Here's how the part is built. I have some questions about the finished solid (model axes, mm). Face numbers are marked on the shaded views. A direction names the side the tool comes from. Give positions to 0.01 mm unless a question says otherwise; leave off trailing zeros. Loops run counter-clockwise (first coordinate to the right, second up) from the corner with the lowest first, then second, coordinate; pieces in that order, holes last. Notation, with made-up numbers: (-15.5, -3.75) - (-2.5, -3.75) arc R36 ccw to (-2.5, 35.25) - close; hole circle Ø1 at (20.25, 40.25). An arc over 180 degrees is marked (long way). One line per item, written item: value. Start each with the question number.
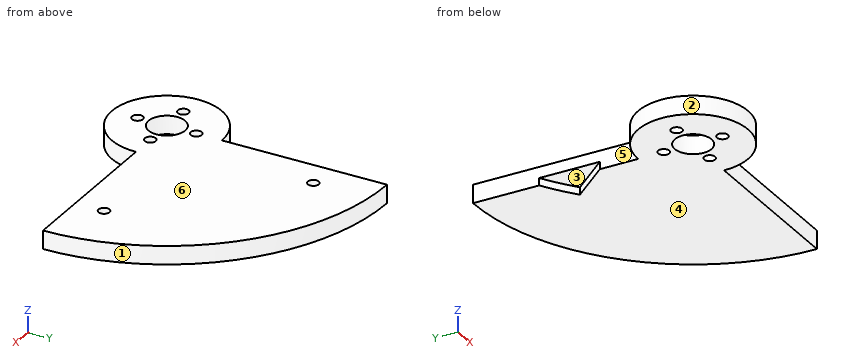
```python
from build123d import *

# Parameters (mm, degrees)
BOSS_EXTRUDE1_DEPTH = 5
SKETCH2_R           = 15
BOSS_EXTRUDE2_DEPTH = 5
SKETCH3_R           = 5
CUT_EXTRUDE1_DEPTH  = 5
SKETCH4_R           = 1.5
CUT_EXTRUDE2_DEPTH  = 2
CUT_EXTRUDE3_DEPTH  = 2
SKETCH6_R           = 1.5
CUT_EXTRUDE4_DEPTH  = 10


with BuildPart() as part:
    # Sketch1 → Boss-Extrude1 (new body)
    with BuildSketch(Plane.XY):
        with BuildLine():
            Line((0, 0), (0, 60))
            ThreePointArc((0, 60), (42.426406871, 42.426406871), (60, 0))
            Line((60, 0), (0, 0))
        make_face()
    extrude(amount=BOSS_EXTRUDE1_DEPTH)

    # Sketch2 → Boss-Extrude2 (add)
    with BuildSketch(Plane.XY.offset(5)):
        Circle(SKETCH2_R)
    extrude(amount=-BOSS_EXTRUDE2_DEPTH)

    # Sketch3 → Cut-Extrude1 (cut)
    with BuildSketch(Plane.XY.offset(5)):
        Circle(SKETCH3_R)
    extrude(amount=-CUT_EXTRUDE1_DEPTH, mode=Mode.SUBTRACT)

    # Sketch4 → Cut-Extrude2 (cut)
    with BuildSketch(Plane.XY.offset(5)):
        with Locations((7.814167995, 44.316348886)):
            Circle(SKETCH4_R)
        with Locations((44.316348886, 7.814167995)):
            Circle(SKETCH4_R)
    extrude(amount=-CUT_EXTRUDE2_DEPTH, mode=Mode.SUBTRACT)

    # Sketch5 → Cut-Extrude3 (cut)
    with BuildSketch(Plane.XY):
        with BuildLine():
            Line((8.772167152, 35.789944904), (-0.110326549, 25.299716292))
            Line((-0.110326549, 25.299716292), (-0.035812461, 41.982184113))
            ThreePointArc((-0.035812461, 41.982184113), (4.507355312, 39.084034363), (8.772167152, 35.789944904))
        make_face()
    extrude(amount=CUT_EXTRUDE3_DEPTH, mode=Mode.SUBTRACT)

    # Sketch6 → Cut-Extrude4 (cut)
    with BuildSketch(Plane.XY.offset(5)):
        with Locations((0, 8)):
            Circle(SKETCH6_R)
        with Locations((8, 0)):
            Circle(SKETCH6_R)
        with Locations((0, -8)):
            Circle(SKETCH6_R)
        with Locations((-8, 0)):
            Circle(SKETCH6_R)
    extrude(amount=-CUT_EXTRUDE4_DEPTH, mode=Mode.SUBTRACT)


solid = part.part
```
(1) Please list where these lines run through material, in increasing order: probe 1 along X at (y, z) = (-1, 0.85); probe 2 along Y at (x, z) = (8, 1.8); probe 3 along Y at (x, z) = (-8, 3). Write a range as from..to.
(2) Will these pins go through, and if not, where does the flat tip stop? pin 1 (1 mm diameter, centred on y = -6, z = 2.5, fed in from +X); pin 2 (1.5 mm diameter, centred on x = 44.5, y = 7.5, fed in from +Z); pin 3 (6 mm diameter, centred on x = 0.5, y = 35, fed in from -Z); pin 4 (2.5 mm diameter, centred on x = 0, y = -8, fed in from -Z).
(3) If we mould it in two halves opening along Y, with no side actions, what happens to the marked faces 1, 2, 3 and 4? For each: pulls with the +Y half, pulls with the -Y half, needs draft (parallel to the pull), parting line crosses it, or undercut.
(4) For the marked faces 5 and 6, which set-ups out of +Z, -Z, +X, -X, +Y, -Y let a thin tool reach every point of the face, with its end or its side?
(5) If we section it at A-A on z = 1: List the corners of the cut face in (x, y) for me, plus the area to 3 significant figures.
(6) If we section it at B-B on x = 7.5: List the corners of the cut face in (y, z) for me.
(7) If we section it at D-D on x = 44: List the corners of the cut face in (y, z) for me.
(8) If we section it at C-C on y = -8: List the corners of the cut face in (x, z) for me, plus the area to 3 significant figures.
Found:
1. probe 1: -14.97..-9.12, -6.88..-4.9, 4.9..6.88, 9.12..14.97
1. probe 2: -12.69..-1.5, 1.5..34.88, 36.43..59.46
1. probe 3: -12.69..-1.5, 1.5..12.69
2. pin 1: x = 13.96
2. pin 2: z = 3
2. pin 3: z = 2
2. pin 4: through
3. face 1: pulls with the +Y half
3. face 2: parting line crosses it
3. face 3: undercut
3. face 4: needs draft
4. face 5: +Z, -Z, -X, +Y
4. face 6: +Z, +X, -X, +Y, -Y
5. outline: (0, 15) arc R15 ccw (long way) to (15, 0) - (60, 0) arc R60 ccw to (0, 60) - (0, 41.96) arc R60 cw to (8.77, 35.79) - (0, 25.43) - close; hole circle Ø3 at (-8, 0); hole circle Ø10 at (0, 0); hole circle Ø3 at (0, -8); hole circle Ø3 at (0, 8); hole circle Ø3 at (8, 0)
5. area: 3,180 mm^2
6. outline: (-12.99, 0) - (-1.41, 0) - (-1.41, 5) - (-12.99, 5) - close; (1.41, 0) - (34.29, 0) - (34.29, 2) - (36.84, 2) - (36.84, 0) - (59.53, 0) - (59.53, 5) - (45.78, 5) - (45.78, 3) - (42.85, 3) - (42.85, 5) - (1.41, 5) - close
7. outline: (0, 0) - (40.79, 0) - (40.79, 5) - (9.28, 5) - (9.28, 3) - (6.35, 3) - (6.35, 5) - (0, 5) - close
8. outline: (-12.69, 0) - (-1.5, 0) - (-1.5, 5) - (-12.69, 5) - close; (1.5, 0) - (12.69, 0) - (12.69, 5) - (1.5, 5) - close
8. area: 112 mm^2
